Geometry: see drawing. Coordinates: mm, zero at the bounding-box minimum. A direction names the side the tool comes from. Coordinates: 2 decimals unless noted, no trailing zeros. Loops run counter-clockwise (first coordinate to the right, second up) from the corner with the lowest first, then second, coordinate; pieces in that order, holes last. Notation, with made-up numbers: M -3,64.25 L 24,64.25 A24 cw 24,101.25 Z; hole C 17.25,15 d1. An arc over 180 degrees is marked long. Write each question's results on one line, items separated by ' | '. Start each with the question number.
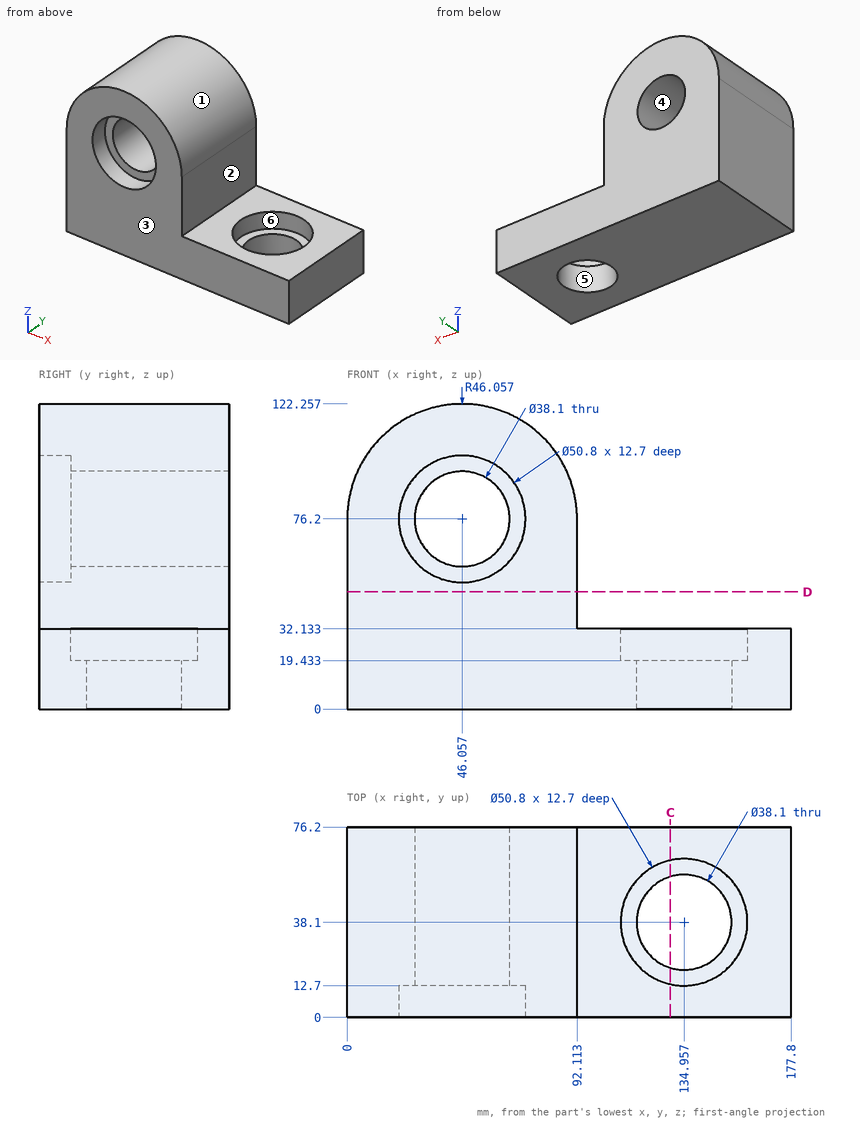
Item 1: First-contact query: pin 1 Ø12 at (x, y) = (73.5, 12) entering from +Z; pin 2 Ø5 at (x, y) = (50.5, 62) entering from +Z; pin 3 Ø6 at (x, z) = (60.5, 74.5) entering from -Y; pin 4 Ø22 at (y, z) = (31.5, 56.5) entering from +X. Flat tips, straight axial feed; report the tip coordinate or a pass-through.
Item 2: Cut plane D-D (z = 47). Output: boundary loops of the cut face in (x, y).
Item 3: Line query: probe 1 along X at (y, z) = (8.5, 77.5) (1 decimal); probe 2 along X at (y, z) = (44, 76) (1 decimal); probe 3 along Z at (x, y) = (60.5, 3.5) (1 decimal). Output: solid intervals per line, ascending.
Item 4: Access query for the marked faces 1 and 2. Directions: +Z, -Z, +X, -X, +Y, -Y. A direction counts if a zero-diameter tool reaches every point of the face in a straight line with its end or side. Return the directions, or none.
Item 5: Mould query, pull axis Y, two halves, no side actions, for the marked faces 3, 4, 5 and 6. Classes: +Y half, -Y half, draft (parallel to the pull), parting line (faces both ways), or undercut.
Item 6: Cut plane C-C (x = 129.5). Output: boundary loops of the cut face in (y, z), then the cut area to 3 significant figures.
Response values:
1) pin 1: stops at z = 116.96 | pin 2: stops at z = 122.22 | pin 3: passes through | pin 4: stops at x = 92.11
2) outline: M 0,0 L 92.11,0 L 92.11,76.2 L 0,76.2 Z
3) probe 1: x = 0 to 20.7, 71.4 to 92.1 | probe 2: x = 0 to 27, 65.1 to 92.1 | probe 3: z = 0 to 55.3, 97.1 to 119.9
4) face 1: +Z, +Y, -Y | face 2: +Z, +X, +Y, -Y
5) face 3: -Y half | face 4: draft | face 5: undercut | face 6: undercut
6) outline: M 0,0 L 19.85,0 L 19.85,19.43 L 13.29,19.43 L 13.29,32.13 L 0,32.13 Z; M 56.35,0 L 76.2,0 L 76.2,32.13 L 62.91,32.13 L 62.91,19.43 L 56.35,19.43 Z | area: 1,110 mm2
